Input: part model. Units: mm. Frame: model coordinates. A direction names the side the tool comes from. Round coordinates to 2 decimals unless told otherwise and drop trailing zeros. One line per question, with ' | ' between items. Start each with the question number.
Q1. Access query for faces 3 (the face through (12.806, 23.79, 1575.592)), 4 (the face through (22.225, 13, 1680)), 5 (the face through (23.835, 11.232, 1791.345)). Directions: +Z, -Z, +X, -X, +Y, -Y. A direction counts if a zero-diameter tool reaches every point of the face in a straight line with its end or side. Return the directions, or none.
Q2. Contact query for flat-ended pins moving along their axis: P1, Ø2, axis at x = 5.5, y = 9, coming from the -Z side; P2, Ø3, axis at x = 3, y = 11.5, coming from the +Z side (3 decimals). Output: stop coordinate, or through.
Q3. Material intervals for L1, parallel to Y at x = 16.25, z = 1751 (3 decimals); L2, parallel to Z at x = 23.5, y = 14, sorted ascending.
Q4. Mould query, pull axis Z, two halves, no side actions, for faces 1 (the face through (13, 0, 1670)), 2 (the face through (12.806, 23.79, 1594.642)). Classes: pulls with the +Z half, pulls with the -Z half, needs draft (parallel to the pull), parting line crosses it, or undercut.
from build123d import *

# Parameters (mm, degrees)
CUT_EXTRUDE1_START = 1516.38
CUT_EXTRUDE1_DEPTH = 312.42
CUT_EXTRUDE2_REACH = 1831.153
CUT_EXTRUDE3_REACH = 1831.153
SKETCH4_R          = 2.413
CUT_EXTRUDE4_DEPTH = 1830.152743759
SKETCH5_R          = 2.413
CUT_EXTRUDE5_DEPTH = 1830.152743759
CUT_EXTRUDE7_REACH = 1831.153
SKETCH8_R          = 2.413


with BuildPart() as part:
    # Cut-Extrude1: read off the stored shape, not the designer's step
    # Cut-Extrude1 outline → Cut-Extrude1 (new body)
    with BuildSketch(Plane.XY.offset(CUT_EXTRUDE1_START)):
        with BuildLine():
            Line((0, 25.146), (0, 0.254))
            ThreePointArc((0, 0.254), (0.074394878, 0.074394878), (0.254, 0))
            Line((0.254, 0), (25.146, 0))
            ThreePointArc((25.146, 0), (25.325605122, 0.074394878), (25.4, 0.254))
            Line((25.4, 0.254), (25.4, 25.146))
            ThreePointArc((25.4, 25.146), (25.325605122, 25.325605122), (25.146, 25.4))
            Line((25.146, 25.4), (0.254, 25.4))
            ThreePointArc((0.254, 25.4), (0.074394878, 25.325605122), (0, 25.146))
        make_face()
        with BuildLine():
            ThreePointArc((4.7625, 3.175), (3.639967985, 3.639967985), (3.175, 4.7625))
            Line((3.175, 4.7625), (3.175, 20.6375))
            ThreePointArc((3.175, 20.6375), (3.639967985, 21.760032015), (4.7625, 22.225))
            Line((4.7625, 22.225), (20.6375, 22.225))
            ThreePointArc((20.6375, 22.225), (21.760032015, 21.760032015), (22.225, 20.6375))
            Line((22.225, 20.6375), (22.225, 4.7625))
            ThreePointArc((22.225, 4.7625), (21.760032015, 3.639967985), (20.6375, 3.175))
            Line((20.6375, 3.175), (4.7625, 3.175))
        make_face(mode=Mode.SUBTRACT)
    extrude(amount=CUT_EXTRUDE1_DEPTH)

    # Cut-Extrude2: up to this face of the body (flat: up to its plane)
    cut_extrude2_end = Plane(part.part.faces().sort_by_distance((12.7, 0, 1672.59))[0])
    # Sketch2 → Cut-Extrude2 (cut, up to the picked face)
    with BuildSketch(Plane(origin=(0, 25.4, 0), x_dir=(1, 0, 0), z_dir=(0, 1, 0)), mode=Mode.PRIVATE) as cut_extrude2_sk1:
        Polygon((43.169380192, -1523.628355708), (25.20886795, -1541.58886795), (-10.712156534, -1505.667843466), (7.248355708, -1487.707331224), align=None)
    cut_extrude2_tool1 = split(extrude(cut_extrude2_sk1.sketch, amount=-CUT_EXTRUDE2_REACH, mode=Mode.PRIVATE), bisect_by=cut_extrude2_end, keep=Keep.BOTH, mode=Mode.PRIVATE)
    add(cut_extrude2_tool1.solids().sort_by(Axis((16.228612, 25.4, 1514.6481), (0, -1, 0)))[0], mode=Mode.SUBTRACT)

    # Cut-Extrude3: up to this face of the body (flat: up to its plane)
    cut_extrude3_end = Plane(part.part.faces().sort_by_distance((12.527724859, 0, 1678.853862429))[0])
    # Sketch3 → Cut-Extrude3 (cut, up to the picked face)
    with BuildSketch(Plane(origin=(0, 25.4, 0), x_dir=(1, 0, 0), z_dir=(0, 1, 0)), mode=Mode.PRIVATE) as cut_extrude3_sk1:
        Polygon((34.192766306, -1837.592766306), (16.232254064, -1855.553278548), (-19.688770421, -1819.632254064), (-1.728258178, -1801.671741822), align=None)
    cut_extrude3_tool1 = split(extrude(cut_extrude3_sk1.sketch, amount=-CUT_EXTRUDE3_REACH, mode=Mode.PRIVATE), bisect_by=cut_extrude3_end, keep=Keep.BOTH, mode=Mode.PRIVATE)
    add(cut_extrude3_tool1.solids().sort_by(Axis((7.251998, 25.4, 1828.61251), (0, -1, 0)))[0], mode=Mode.SUBTRACT)

    # Sketch4 → Cut-Extrude4 (cut, through all)
    with BuildSketch(Plane(origin=(0, 25.4, 0), x_dir=(1, 0, 0), z_dir=(0, 1, 0))):
        with Locations(Location((12.7, -1789.159231637, 0), (0, 0, 270))):
            Circle(SKETCH4_R)
        with Locations(Location((12.7, -1712.959231637, 0), (0, 0, 270))):
            Circle(SKETCH4_R)
        with Locations(Location((12.7, -1636.759231637, 0), (0, 0, 270))):
            Circle(SKETCH4_R)
    extrude(amount=-CUT_EXTRUDE4_DEPTH, mode=Mode.SUBTRACT)

    # Sketch5 → Cut-Extrude5 (cut, through all)
    with BuildSketch(Plane.XZ):
        with Locations(Location((7.439487758, 1541.431804126, 0), (0, 0, 270))):
            Circle(SKETCH5_R)
        with Locations(Location((12.7, 1554.131804126, 0), (0, 0, 270))):
            Circle(SKETCH5_R)
        with Locations(Location((12.7, 1573.181804126, 0), (0, 0, 270))):
            Circle(SKETCH5_R)
        with Locations(Location((12.7, 1592.231804126, 0), (0, 0, 270))):
            Circle(SKETCH5_R)
    extrude(amount=-CUT_EXTRUDE5_DEPTH, mode=Mode.SUBTRACT)

    # Sketch8 → Cut-Extrude7 (cut, up to next)
    with BuildSketch(Plane(origin=(25.4, 0, 0), x_dir=(0, 0, -1), z_dir=(1, 0, 0)), mode=Mode.PRIVATE) as cut_extrude7_sk1:
        with Locations((-1814.83, 12.7)):
            Circle(SKETCH8_R)
    cut_extrude7_tool1 = extrude(cut_extrude7_sk1.sketch, amount=-CUT_EXTRUDE7_REACH, mode=Mode.PRIVATE) & part.part
    # Sketch8 → Cut-Extrude7 (cut, up to next)
    with BuildSketch(Plane(origin=(25.4, 0, 0), x_dir=(0, 0, -1), z_dir=(1, 0, 0)), mode=Mode.PRIVATE) as cut_extrude7_sk2:
        with Locations((-1789.43, 12.7)):
            Circle(SKETCH8_R)
    cut_extrude7_tool2 = extrude(cut_extrude7_sk2.sketch, amount=-CUT_EXTRUDE7_REACH, mode=Mode.PRIVATE) & part.part
    add(cut_extrude7_tool1.solids().sort_by_distance((25.4, 12.7, 1814.83))[0], mode=Mode.SUBTRACT)
    add(cut_extrude7_tool2.solids().sort_by_distance((25.4, 12.7, 1789.43))[0], mode=Mode.SUBTRACT)


solid = part.part
Results:
1) face 3: +Y, -Y | face 4: +Z, -Z | face 5: +X
2) P1: through | P2: z = 1806.575
3) L1: 0 to 3.175, 22.225 to 25.4 | L2: 1539.88 to 1787.4, 1791.46 to 1812.8, 1816.86 to 1826.9
4) face 1: needs draft | face 2: undercut
